Could you check a few things on this model? Use its own coordinates, in mm. A direction names the side the tool comes from. Coordinates: 2 decimals unless noted, no trailing zeros.
1) For faces 5 (the face through (18.07, 17, 7)), 6 (the face through (39, 5, 0)), 7 (the face through (5.58, 30.2, 11.57)), which set-ups out of +Z, -Z, +X, -X, +Y, -Y let a thin tool reach every point of the face, with its end or its side?
2) If I drill on line 1 along X through (y, z) = (20, -9.5); line 2 along Y through (x, z) = (6, -3.5); line 3 along X through (y, z) = (3, 0), over which ranges is the centre line in solid material (lowest first)?
3) Will these pins go through, and if not, where does the flat tip stop? P1, Ø6, axis at y = 25, z = -7.5, coming from the +X side; P2, Ø17, axis at x = 31.5, y = 16.5, coming from the -Z side; P3, Ø2, axis at y = 29, z = 0.5, coming from the +X side.
4) Thinking about a two-plate mould opening in X: for faces 1 (the face through (27, 19, -1.5)), 2 (the face through (-47.15, 2.46, 16.99)), 3 (the face through (-10.42, 35.01, -4.83)), 4 (the face through (50, 2, 0)), which applies, released by +X, released by -X, zero draft, split by the parting line, or undercut?
```python
from build123d import *

# Parameters (mm, degrees)
BOSS_EXTRUDE1_DEPTH = 5
BOSS_EXTRUDE2_REACH = 98.884
SKETCH2_R           = 15
SKETCH2_R_2         = 12.5
BOSS_EXTRUDE3_REACH = 98.884
SKETCH3_R           = 1
RIB1_REACH          = 87.478
SKETCH4_WALL_W      = 198.83792102
SKETCH4_WALL_H      = 3
RIB2_REACH          = 100.216
SKETCH5_WALL_W      = 242.211652072
SKETCH5_WALL_H      = 3
SKETCH6_R           = 1.5
CUT_EXTRUDE1_DEPTH  = 5


with BuildPart() as part:
    # Sketch1 → Boss-Extrude1 (new body)
    with BuildSketch(Plane(origin=(0, 0, 0), x_dir=(1, 0, 0), z_dir=(0, 1, 0))):
        with BuildLine():
            Line((40, 20), (-40, 20))
            ThreePointArc((-40, 20), (-47.071067812, 17.071067812), (-50, 10))
            Line((-50, 10), (-50, -10))
            ThreePointArc((-50, -10), (-47.071067812, -17.071067812), (-40, -20))
            Line((-40, -20), (40, -20))
            ThreePointArc((40, -20), (47.071067812, -17.071067812), (50, -10))
            Line((50, -10), (50, 10))
            ThreePointArc((50, 10), (47.071067812, 17.071067812), (40, 20))
        make_face()
    extrude(amount=BOSS_EXTRUDE1_DEPTH)

    # Boss-Extrude2: up to this plane
    boss_extrude2_end = Plane(origin=(40, 5, 10), z_dir=(0, -1, 0))
    # Sketch2 → Boss-Extrude2 (add, up to the surface)
    with BuildSketch(Plane(origin=(29.665063509, 51.381397208, 0), x_dir=(0, 0, -1), z_dir=(0.500000000000001, 0.866025403784438, 0)), mode=Mode.PRIVATE) as boss_extrude2_sk1:
        with Locations(Location((0, 15, 0), (0, 0, 90))):
            Circle(SKETCH2_R)
        with Locations(Location((0, 15, 0), (0, 0, 90))):
            Circle(SKETCH2_R_2, mode=Mode.SUBTRACT)
    boss_extrude2_tool1 = split(extrude(boss_extrude2_sk1.sketch, amount=-BOSS_EXTRUDE2_REACH, mode=Mode.PRIVATE), bisect_by=boss_extrude2_end, keep=Keep.BOTH, mode=Mode.PRIVATE)
    add(boss_extrude2_tool1.solids().sort_by_distance((29.29764, 51.593529, 0))[0])

    # Boss-Extrude3: up to this plane
    boss_extrude3_end = Plane(origin=(40, 5, 10), z_dir=(0, -1, 0))
    # Sketch3 → Boss-Extrude3 (add, up to the surface)
    with BuildSketch(Plane(origin=(29.665063509, 51.381397208, 0), x_dir=(0.8660254037844382, -0.500000000000001, 0), z_dir=(0.500000000000001, 0.8660254037844382, 0)), mode=Mode.PRIVATE) as boss_extrude3_sk1:
        with Locations((-2.5, 0)):
            Circle(SKETCH3_R)
    boss_extrude3_tool1 = split(extrude(boss_extrude3_sk1.sketch, amount=-BOSS_EXTRUDE3_REACH, mode=Mode.PRIVATE), bisect_by=boss_extrude3_end, keep=Keep.BOTH, mode=Mode.PRIVATE)
    add(boss_extrude3_tool1.solids().sort_by_distance((27.5, 52.631397, 0))[0])
    # Sketch3 → Boss-Extrude3 (add, up to the surface)
    with BuildSketch(Plane(origin=(29.665063509, 51.381397208, 0), x_dir=(0.8660254037844382, -0.500000000000001, 0), z_dir=(0.500000000000001, 0.8660254037844382, 0)), mode=Mode.PRIVATE) as boss_extrude3_sk2:
        with Locations((-6.161165235, -8.838834765)):
            Circle(SKETCH3_R)
    boss_extrude3_tool2 = split(extrude(boss_extrude3_sk2.sketch, amount=-BOSS_EXTRUDE3_REACH, mode=Mode.PRIVATE), bisect_by=boss_extrude3_end, keep=Keep.BOTH, mode=Mode.PRIVATE)
    add(boss_extrude3_tool2.solids().sort_by_distance((24.329338, 54.46198, 8.838835))[0])
    # Sketch3 → Boss-Extrude3 (add, up to the surface)
    with BuildSketch(Plane(origin=(29.665063509, 51.381397208, 0), x_dir=(0.8660254037844382, -0.500000000000001, 0), z_dir=(0.500000000000001, 0.8660254037844382, 0)), mode=Mode.PRIVATE) as boss_extrude3_sk3:
        with Locations((-15, -12.5)):
            Circle(SKETCH3_R)
    boss_extrude3_tool3 = split(extrude(boss_extrude3_sk3.sketch, amount=-BOSS_EXTRUDE3_REACH, mode=Mode.PRIVATE), bisect_by=boss_extrude3_end, keep=Keep.BOTH, mode=Mode.PRIVATE)
    add(boss_extrude3_tool3.solids().sort_by_distance((16.674682, 58.881397, 12.5))[0])
    # Sketch3 → Boss-Extrude3 (add, up to the surface)
    with BuildSketch(Plane(origin=(29.665063509, 51.381397208, 0), x_dir=(0.8660254037844382, -0.500000000000001, 0), z_dir=(0.500000000000001, 0.8660254037844382, 0)), mode=Mode.PRIVATE) as boss_extrude3_sk4:
        with Locations((-23.838834765, -8.838834765)):
            Circle(SKETCH3_R)
    boss_extrude3_tool4 = split(extrude(boss_extrude3_sk4.sketch, amount=-BOSS_EXTRUDE3_REACH, mode=Mode.PRIVATE), bisect_by=boss_extrude3_end, keep=Keep.BOTH, mode=Mode.PRIVATE)
    add(boss_extrude3_tool4.solids().sort_by_distance((9.020027, 63.300815, 8.838835))[0])
    # Sketch3 → Boss-Extrude3 (add, up to the surface)
    with BuildSketch(Plane(origin=(29.665063509, 51.381397208, 0), x_dir=(0.8660254037844382, -0.500000000000001, 0), z_dir=(0.500000000000001, 0.8660254037844382, 0)), mode=Mode.PRIVATE) as boss_extrude3_sk5:
        with Locations((-27.5, 0)):
            Circle(SKETCH3_R)
    boss_extrude3_tool5 = split(extrude(boss_extrude3_sk5.sketch, amount=-BOSS_EXTRUDE3_REACH, mode=Mode.PRIVATE), bisect_by=boss_extrude3_end, keep=Keep.BOTH, mode=Mode.PRIVATE)
    add(boss_extrude3_tool5.solids().sort_by_distance((5.849365, 65.131397, 0))[0])
    # Sketch3 → Boss-Extrude3 (add, up to the surface)
    with BuildSketch(Plane(origin=(29.665063509, 51.381397208, 0), x_dir=(0.8660254037844382, -0.500000000000001, 0), z_dir=(0.500000000000001, 0.8660254037844382, 0)), mode=Mode.PRIVATE) as boss_extrude3_sk6:
        with Locations((-23.838834765, 8.838834765)):
            Circle(SKETCH3_R)
    boss_extrude3_tool6 = split(extrude(boss_extrude3_sk6.sketch, amount=-BOSS_EXTRUDE3_REACH, mode=Mode.PRIVATE), bisect_by=boss_extrude3_end, keep=Keep.BOTH, mode=Mode.PRIVATE)
    add(boss_extrude3_tool6.solids().sort_by_distance((9.020027, 63.300815, -8.838835))[0])
    # Sketch3 → Boss-Extrude3 (add, up to the surface)
    with BuildSketch(Plane(origin=(29.665063509, 51.381397208, 0), x_dir=(0.8660254037844382, -0.500000000000001, 0), z_dir=(0.500000000000001, 0.8660254037844382, 0)), mode=Mode.PRIVATE) as boss_extrude3_sk7:
        with Locations((-15, 12.5)):
            Circle(SKETCH3_R)
    boss_extrude3_tool7 = split(extrude(boss_extrude3_sk7.sketch, amount=-BOSS_EXTRUDE3_REACH, mode=Mode.PRIVATE), bisect_by=boss_extrude3_end, keep=Keep.BOTH, mode=Mode.PRIVATE)
    add(boss_extrude3_tool7.solids().sort_by_distance((16.674682, 58.881397, -12.5))[0])
    # Sketch3 → Boss-Extrude3 (add, up to the surface)
    with BuildSketch(Plane(origin=(29.665063509, 51.381397208, 0), x_dir=(0.8660254037844382, -0.500000000000001, 0), z_dir=(0.500000000000001, 0.8660254037844382, 0)), mode=Mode.PRIVATE) as boss_extrude3_sk8:
        with Locations((-6.161165235, 8.838834765)):
            Circle(SKETCH3_R)
    boss_extrude3_tool8 = split(extrude(boss_extrude3_sk8.sketch, amount=-BOSS_EXTRUDE3_REACH, mode=Mode.PRIVATE), bisect_by=boss_extrude3_end, keep=Keep.BOTH, mode=Mode.PRIVATE)
    add(boss_extrude3_tool8.solids().sort_by_distance((24.329338, 54.46198, -8.838835))[0])

    # Sketch4 wall → Rib1 (add, up to next)
    with BuildSketch(Plane(origin=(31.650635095, 22.5, 0), x_dir=(0.258819045111, -0.965925826287, 0), z_dir=(0.965925826287, 0.258819045111, 0)), mode=Mode.PRIVATE) as rib1_sk1:
        Rectangle(SKETCH4_WALL_W, SKETCH4_WALL_H)
    rib1_tool1 = extrude(rib1_sk1.sketch, amount=-RIB1_REACH, mode=Mode.PRIVATE) - part.part
    add(rib1_tool1.solids().sort_by_distance((31.650635095, 22.5, 0))[0])

    # Sketch5 wall → Rib2 (add, up to next)
    with BuildSketch(Plane(origin=(19.569838586, 24.839013436, 10.75), x_dir=(0, -0.906326752135, 0.422577588573), z_dir=(0, -0.422577588573, -0.906326752135)), mode=Mode.PRIVATE) as rib2_sk1:
        Rectangle(SKETCH5_WALL_W, SKETCH5_WALL_H)
    rib2_tool1 = extrude(rib2_sk1.sketch, amount=RIB2_REACH, mode=Mode.PRIVATE) - part.part
    rib2 = rib2_tool1.solids().sort_by_distance((19.569838586, 24.839013436, 10.75))[0]
    add(rib2)

    # Mirror2: Rib2 across plane
    add(rib2.mirror(Plane.XY))

    # Sketch6 → Cut-Extrude1 (cut)
    with BuildSketch(Plane(origin=(0, 0, 0), x_dir=(-1, 0, 0), z_dir=(0, -1, 0))):
        with Locations(Location((-40, 15, 0), (0, 0, 90))):
            Circle(SKETCH6_R)
        with Locations(Location((-40, -15, 0), (0, 0, 90))):
            Circle(SKETCH6_R)
        with Locations(Location((40, 0, 0), (0, 0, 90))):
            Circle(SKETCH6_R)
    extrude(amount=-CUT_EXTRUDE1_DEPTH, mode=Mode.SUBTRACT)


solid = part.part
```
Filled in:
1. face 5: +Z
1. face 6: +X
1. face 7: none
2. line 1: x = -19.18 to -15.11, 3.57 to 7.63, 18.07 to 21.07
2. line 2: y = 0 to 5, 11.22 to 16.39, 64.39 to 65.04
2. line 3: x = -50 to -41.5, -38.5 to 50
3. P1: stops at x = 21.07
3. P2: stops at z = -1.5
3. P3: stops at x = 30.18
4. face 1: zero draft
4. face 2: released by -X
4. face 3: undercut
4. face 4: released by +X
